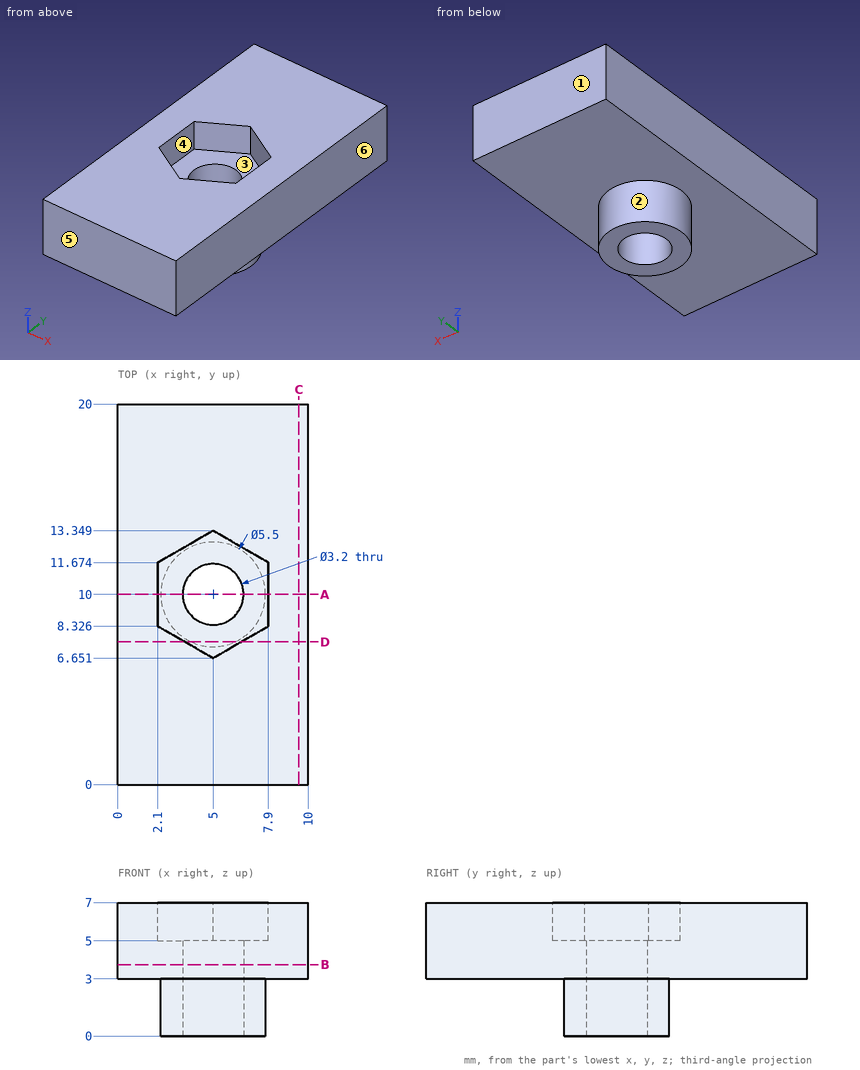
Design review of the part shown in the three views and the two pictorial views. Dimensions are in mm from the part's minimum x, y and z. A direction names the side the tool comes from. Round coordinates to 2 decimals unless told otherwise and drop trailing zeros. Write each loop counter-clockwise with the first axis right and the second up, starting at its lowest first coordinate (ties: lowest second). Pieces come first, ordered by that corner, then holes. Notation, with made-up numbers: (68.5, 64) - (112.5, 64) arc R26 cw to (112.5, 91) - close; hole circle Ø7 at (22, 52.25). An arc over 180 degrees is marked (long way). Return JSON: item names as keys, results as strings. Group by question number.
Item 1: We need section A-A on y = 10. Write out the cut boundary in (x, z).
Item 2: We need section C-C on x = 9.5. Write out the cut boundary in (y, z), and give its area (3 significant figures).
Item 3: We need section B-B on z = 3.75. Write out the cut boundary in (x, y).
Item 4: Insertion check: P1, Ø4.5, axis at x = 4.5, y = 10, coming from the +Z side; P2, Ø2, axis at x = 2.5, y = 5, coming from the -Z side. Each pin has a flat end and moves straight along its axis. Give the tip position at first contact, or say it passes through.
Item 5: The part is to be moulded in two halves that separate along Y. For the marked faces 4, 5 and 6, say which applies: pulls with the +Y half, pulls with the -Y half, needs draft (parallel to the pull), parting line crosses it, or undercut.
Item 6: Machinability: for the marked faces 1, 2 and 3, which of the approach directions +Z, -Z, +X, -X, +Y, -Y give a long, thin tool a straight path to every point of the face, cutting with its end or side? Answer none if there is none.
Item 7: For probe 1 along Y at (x, z) = (5, 3.8); probe 2 along X at (y, z) = (11.5, 6.25); probe 3 along Z at (x, y) = (2.5, 13.25), list the stretches that pass through material, from the lowest coordinate up. Write a range as [from, to].
Item 8: We need section D-D on y = 7.5. Write out the cut boundary in (x, z) (1 decimal).
Model answer:
{
 "1": {"outline": "(0, 3) - (2.25, 3) - (2.25, 0) - (3.4, 0) - (3.4, 5) - (2.1, 5) - (2.1, 7) - (0, 7) - close; (6.6, 0) - (7.75, 0) - (7.75, 3) - (10, 3) - (10, 7) - (7.9, 7) - (7.9, 5) - (6.6, 5) - close"},
 "2": {"outline": "(0, 3) - (20, 3) - (20, 7) - (0, 7) - close", "area": "80.0 mm²"},
 "3": {"outline": "(0, 0) - (10, 0) - (10, 20) - (0, 20) - close; hole circle Ø3.2 at (5, 10)"},
 "4": {"P1": "stops at z = 5", "P2": "stops at z = 3"},
 "5": {"face 4": "undercut", "face 5": "pulls with the -Y half", "face 6": "needs draft"},
 "6": {"face 1": "+Z, -Z, +X, -X, +Y", "face 2": "-Z", "face 3": "+Z"},
 "7": {"probe 1": "y = [0, 8.4], [11.6, 20]", "probe 2": "x = [0, 2.1], [7.9, 10]", "probe 3": "z = [3, 7]"},
 "8": {"outline": "(0, 3) - (3.9, 3) - (3.9, 0) - (6.1, 0) - (6.1, 3) - (10, 3) - (10, 7) - (6.5, 7) - (6.5, 5) - (3.5, 5) - (3.5, 7) - (0, 7) - close"}
}
